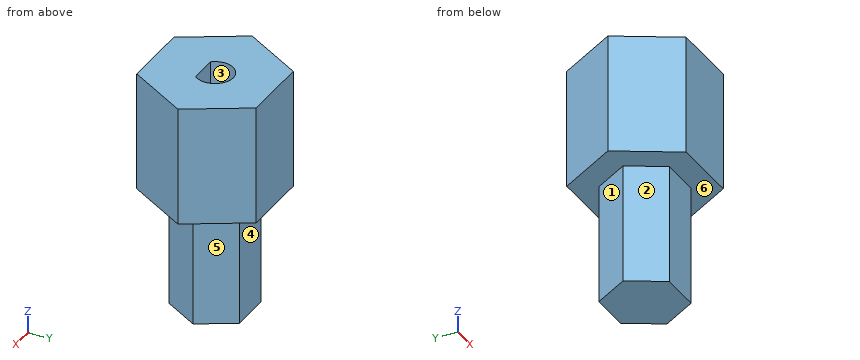
from build123d import *

# Parameters (mm, degrees)
BOSS_EXTRUDE1_DEPTH = 20
BOSS_EXTRUDE2_DEPTH = 10
CUT_EXTRUDE1_DEPTH  = 11


with BuildPart() as part:
    # Sketch1 → Boss-Extrude1 (new body)
    with BuildSketch(Plane.XY):
        Polygon((3.406366588, 0), (1.703183294, 2.95), (-1.703183294, 2.95), (-3.406366588, 0), (-1.703183294, -2.95), (1.703183294, -2.95), align=None)
    extrude(amount=BOSS_EXTRUDE1_DEPTH)

    # Sketch2 → Boss-Extrude2 (add)
    with BuildSketch(Plane.XY.offset(20)):
        Polygon((-5.773502692, 0), (-2.886751346, -5), (2.886751346, -5), (5.773502692, 0), (2.886751346, 5), (-2.886751346, 5), align=None)
    extrude(amount=-BOSS_EXTRUDE2_DEPTH)

    # Sketch4 → Cut-Extrude1 (cut)
    with BuildSketch(Plane.XY.offset(20)):
        with BuildLine():
            Line((-1.157972366, -1), (1.157972366, -1))
            ThreePointArc((1.157972366, -1), (0, 1.53), (-1.157972366, -1))
        make_face()
    extrude(amount=-CUT_EXTRUDE1_DEPTH, mode=Mode.SUBTRACT)


solid = part.part
The model under review builds one solid part; all positions refer to its coordinate system, in mm. Face numbers are marked on the shaded views. A direction names the side the tool comes from. Coordinates: 2 decimals unless noted, no trailing zeros. Write each loop counter-clockwise with the first axis right and the second up, starting at its lowest first coordinate (ties: lowest second). Pieces come first, ordered by that corner, then holes. Notation, with made-up numbers: (1.5, 70.25) - (15.5, 70.25) arc R29 cw to (15.5, 106.25) - close; hole circle Ø5 at (83, 3.25). An arc over 180 degrees is marked (long way). Answer as a JSON object with one key per item and string values. Group by question number.
1. Machinability: for the marked faces 4, 5 and 6, which of the approach directions +Z, -Z, +X, -X, +Y, -Y give a long, thin tool a straight path to every point of the face, cutting with its end or side? Answer none if there is none.
2. Add section A-A (z = 12.25). Give the boundary of the cut face in (x, y), plus the area to 3 significant figures.
3. Add section B-B (x = 0). Give the boundary of the cut face in (y, z).
4. To check wall thickness, follow probe 1 along Y at (x, z) = (0, 16); probe 2 along Z at (x, y) = (-4, -3); probe 3 along X at (y, z) = (-1.75, 1). State the ranges of each line that lie inside material, in increasing order.
5. Add section D-D (z = 8.5). Give the boundary of the cut face in (x, y), plus the area to 3 significant figures.
6. Clearance check with flat-ended pins moving along their axes: pin 1 Ø0.8 at (x, y) = (0.5, 0.5) entering from +Z; pin 2 Ø1 at (y, z) = (-3.5, 11) entering from -X; pin 3 Ø2.5 at (x, y) = (0, 0) entering from -Z; pin 4 Ø5 at (x, z) = (-4, 6.5) entering from +Y. State where each tip first meets the part, or that it passes through.
7. Mouldability with a two-part tool opening along Y and no side actions: class the marked faces 1, 2 and 3 as pulls with the +Y half, pulls with the -Y half, needs draft (parallel to the pull), parting line crosses it, or undercut.
8. Add section C-C (y = 1). Give the boundary of the cut face in (x, z).
Findings:
{
 "1": {"face 4": "-Z, +X, -X, +Y", "face 5": "-Z, +X, +Y", "face 6": "-Z"},
 "2": {"outline": "(-5.77, 0) - (-2.89, -5) - (2.89, -5) - (5.77, 0) - (2.89, 5) - (-2.89, 5) - close; hole (-1.16, -1) - (1.16, -1) arc R1.53 ccw (long way) to start", "area": "80.1 mm²"},
 "3": {"outline": "(-5, 10) - (-2.95, 10) - (-2.95, 0) - (2.95, 0) - (2.95, 10) - (5, 10) - (5, 20) - (1.53, 20) - (1.53, 9) - (-1, 9) - (-1, 20) - (-5, 20) - close"},
 "4": {"probe 1": "-5 to -1, 1.53 to 5", "probe 2": "10 to 20", "probe 3": "-2.4 to 2.4"},
 "5": {"outline": "(-3.41, 0) - (-1.7, -2.95) - (1.7, -2.95) - (3.41, 0) - (1.7, 2.95) - (-1.7, 2.95) - close", "area": "30.1 mm²"},
 "6": {"pin 1": "z = 9", "pin 2": "x = -4.04", "pin 3": "z = 0", "pin 4": "y = 2.95"},
 "7": {"face 1": "pulls with the +Y half", "face 2": "pulls with the -Y half", "face 3": "undercut"},
 "8": {"outline": "(-5.2, 10) - (-2.83, 10) - (-2.83, 0) - (2.83, 0) - (2.83, 10) - (5.2, 10) - (5.2, 20) - (1.16, 20) - (1.16, 9) - (-1.16, 9) - (-1.16, 20) - (-5.2, 20) - close"}
}
